from build123d import *

# Parameters (mm, degrees)
SKETCH1_R           = 2228.848425932
SKETCH1_R_2         = 2232.515095695
SKETCH1_R_3         = 2255.383637046
SKETCH1_R_4         = 2221.194192251
SKETCH1_R_5         = 2229.264638927
SKETCH1_R_6         = 2222.153252204
SKETCH1_R_7         = 2227.962328558
SKETCH1_R_8         = 2234.328555728
BOSS_EXTRUDE1_DEPTH = 3500
SKETCH2_W           = 61968.445691345
SKETCH2_H           = 92600
BOSS_EXTRUDE2_DEPTH = 20000
SCALE1_SCALE        = 0.001


with BuildPart() as part:
    # Sketch1 → Boss-Extrude1 (new body)
    with BuildSketch(Plane.XY):
        with BuildLine():
            ThreePointArc((106545.079885482, 100518.436826227), (106853.327609477, 105879.024620733), (101661.548830659, 107248.824341048))
            ThreePointArc((101661.548830659, 107248.824341048), (53788.50438499, 96874.393209157), (5922.956321239, 107283.35638346))
            ThreePointArc((5922.956321239, 107283.35638346), (817.61837842, 105942.536812531), (1110.36774195, 100672.188584726))
            ThreePointArc((1110.36774195, 100672.188584726), (19271.211317967, 53879.37747984), (1130.518180486, 7078.750742777))
            ThreePointArc((1130.518180486, 7078.750742777), (546.608093922, 2206.067347313), (4967.687443421, 75.796977839))
            ThreePointArc((4967.687443421, 75.796977839), (53840.129347423, 4274.393209157), (102711.67644046, 65.394194326))
            ThreePointArc((102711.67644046, 65.394194326), (107170.596097397, 2217.573525566), (106569.543420865, 7132.100569023))
            ThreePointArc((106569.543420865, 7132.100569023), (88370.47645447, 53820.504464396), (106545.079885482, 100518.436826227))
        make_face()
        with Locations((103434.821241174, 103424.132598226)):
            Circle(SKETCH1_R, mode=Mode.SUBTRACT)
        with Locations((4216.199864712, 103431.93144758)):
            Circle(SKETCH1_R_2, mode=Mode.SUBTRACT)
        with Locations((4214.875121526, 4248.849141113)):
            Circle(SKETCH1_R_3, mode=Mode.SUBTRACT)
        with Locations((103411.028421454, 4238.866596861)):
            Circle(SKETCH1_R_4, mode=Mode.SUBTRACT)
        with Locations((91025.969819716, 16629.576138342)):
            Circle(SKETCH1_R_5, mode=Mode.SUBTRACT)
        with Locations((16598.170941579, 16611.164460881)):
            Circle(SKETCH1_R_6, mode=Mode.SUBTRACT)
        with Locations((16610.109502545, 91032.533832428)):
            Circle(SKETCH1_R_7, mode=Mode.SUBTRACT)
        with Locations((91028.833016767, 91029.045185522)):
            Circle(SKETCH1_R_8, mode=Mode.SUBTRACT)
    extrude(amount=BOSS_EXTRUDE1_DEPTH)

    # Sketch2 → Boss-Extrude2 (add)
    with BuildSketch(Plane.XY.offset(3500)):
        with Locations((53840.129347424, 50574.393209157)):
            Rectangle(SKETCH2_W, SKETCH2_H)
    extrude(amount=BOSS_EXTRUDE2_DEPTH)


with BuildPart() as part_1:
    # Scale1: scaled about (53841.453243905, 50705.922203797, 11214.696487876)
    add(part.part.scale(SCALE1_SCALE).moved(Location((53787.611790661, 50655.216281593, 11203.481791388))))


solid = part_1.part
CAD build for the part. Positions are in the model's coordinates, mm. A direction names the side the tool comes from. Round coordinates to 2 decimals unless told otherwise and drop trailing zeros. Write each loop counter-clockwise with the first axis right and the second up, starting at its lowest first coordinate (ties: lowest second). Pieces come first, ordered by that corner, then holes.
(1) Slice it at D-D, the plane x = 53866. Write the cut outline in (y, z).
(2) 3-axis set-ups, long thin cutter, end or side, ignore diameter. For faces 5 (the face through (53791.338, 50657.263, 11205.207)), 6 (the face through (53841, 50752.091, 11217)), 7 (the face through (53872.436, 50705, 11217)), 8 (the face through (53841, 50659.491, 11217)): which of +Z, -Z, +X, -X, +Y, -Y reach the whole face in a straight line?
(3) Drop flat-ended pins along their axis: P1, Ø1.5, axis at y = 50669.5, z = 11219.5, coming from the +X side; P2, Ø6, axis at x = 53791.83, y = 50659.47, coming from the -Z side; P3, Ø1, axis at y = 50696.5, z = 11210.5, coming from the -X side; P4, Ø10, axis at x = 53843.5, z = 11220.5, coming from the +Y side. Give the stop position or say it passes through.
(4) Slice it at B-B, the plane x = 53882.5. Write the cut outline in (y, z), and give its area (3 significant figures).
(5) Probe line 1 along X through (y, z) = (50750, 11210.5); line 2 along Y through (x, z) = (53830, 11216.75); line 3 along X through (y, z) = (50709, 11204.75). List the from-to ranges inside material, lowest first.
(6) Slice it at C-C, the plane y = 50668. Write the cut outline in (x, z).
(7) Slice it at A-A, the plane z = 11205. Count the separate pieces of the cut face and the enclosed holes in it, and give its area (3 significant figures).
(8) Mould opens along X. For faces 1 (the face through (53841, 50706, 11226.982)), 2 (the face through (53875.986, 50708.319, 11205.207)), 3 (the face through (53840.76, 50659.49, 11205.21)), 4 (the face through (53810.468, 50705, 11217)) say: pulls with the +X half, pulls with the -X half, needs draft (parallel to the pull), parting line crosses it, or undercut.
From the geometry:
1. outline: (50658.43, 11203.48) - (50754.73, 11203.48) - (50754.73, 11206.98) - (50752.09, 11206.98) - (50752.09, 11226.98) - (50659.49, 11226.98) - (50659.49, 11206.98) - (50658.43, 11206.98) - close
2. face 5: +Z, -Z
2. face 6: +Z, +X, -X, +Y
2. face 7: +Z, +X, +Y, -Y
2. face 8: +Z, +X, -X, -Y
3. P1: stops at x = 53872.44
3. P2: stops at z = 11203.48
3. P3: stops at x = 53810.47
3. P4: stops at y = 50752.09
4. outline: (50656.53, 11203.48) - (50679.77, 11203.48) - (50679.77, 11206.98) - (50656.53, 11206.98) - close; (50738.34, 11203.48) - (50759.64, 11203.48) - (50759.64, 11206.98) - (50738.34, 11206.98) - close
4. area: 156 mm2
5. line 1: x = 53810.47 to 53872.44
5. line 2: y = 50659.49 to 50752.09
5. line 3: x = 53806.88 to 53875.98
6. outline: (53793.42, 11203.48) - (53889.52, 11203.48) - (53889.52, 11206.98) - (53872.44, 11206.98) - (53872.44, 11226.98) - (53810.47, 11226.98) - (53810.47, 11206.98) - (53793.42, 11206.98) - close
7. separate pieces: 1
7. enclosed holes: 8
7. area: 7,920 mm2
8. face 1: needs draft
8. face 2: pulls with the +X half
8. face 3: undercut
8. face 4: pulls with the -X half
